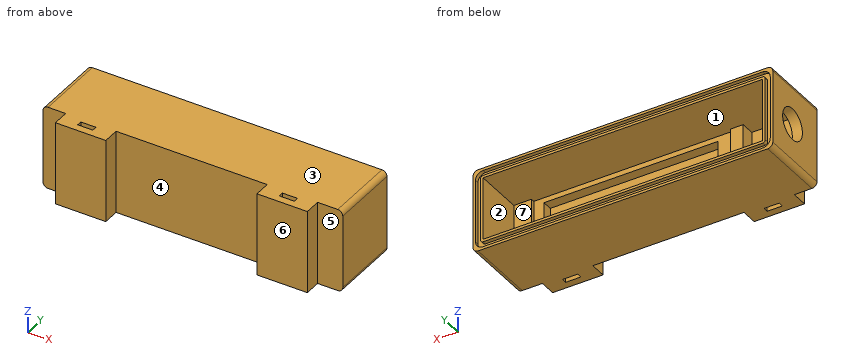
from build123d import *

# Parameters (mm, degrees)
SZKIC5_W                    = 119
SZKIC5_H                    = 33
DODANIE_WYCI_GNI_CIE3_DEPTH = 3
SZKIC6_W                    = 119
SZKIC6_H                    = 33
SZKIC6_W_2                  = 111
SZKIC6_H_2                  = 25
DODANIE_WYCI_GNI_CIE4_DEPTH = 25
SZKIC7_W                    = 91
SZKIC7_H                    = 25
SZKIC7_W_2                  = 69
SZKIC7_H_2                  = 21
DODANIE_WYCI_GNI_CIE5_DEPTH = 4
SZKIC8_W                    = 5
SZKIC8_H                    = 25
SZKIC8_W_2                  = 7
DODANIE_WYCI_GNI_CIE6_DEPTH = 1.5
SZKIC10_R                   = 6.25
WYTNIJ_WYCI_GNI_CIE1_DEPTH  = 7.5
SZKIC22_W                   = 2
SZKIC22_H                   = 3
BOSS_EXTRUDE2_DEPTH         = 20
FILLET1_R                   = 2
SKETCH2_W                   = 6
SKETCH2_H                   = 2
CUT_EXTRUDE1_DEPTH          = 33
FILLET2_R                   = 2
FILLET3_R                   = 2
CUT_EXTRUDE2_DEPTH          = 111


with BuildPart() as part:
    # Szkic5 → Dodanie-wyciągnięcie3 (new body)
    with BuildSketch(Plane(origin=(0, 0, 0), x_dir=(1, 0, 0), z_dir=(0, 1, 0))):
        Rectangle(SZKIC5_W, SZKIC5_H)
    extrude(amount=DODANIE_WYCI_GNI_CIE3_DEPTH)

    # Szkic6 → Dodanie-wyciągnięcie4 (add)
    with BuildSketch(Plane(origin=(0, 3, 0), x_dir=(1, 0, 0), z_dir=(0, 1, 0))):
        Rectangle(SZKIC6_W, SZKIC6_H)
        Rectangle(SZKIC6_W_2, SZKIC6_H_2, mode=Mode.SUBTRACT)
    extrude(amount=DODANIE_WYCI_GNI_CIE4_DEPTH)

    # Szkic7 → Dodanie-wyciągnięcie5 (add)
    with BuildSketch(Plane(origin=(0, 3, 0), x_dir=(1, 0, 0), z_dir=(0, 1, 0))):
        with Locations((10, 0)):
            Rectangle(SZKIC7_W, SZKIC7_H)
        with Locations((10, 0)):
            Rectangle(SZKIC7_W_2, SZKIC7_H_2, mode=Mode.SUBTRACT)
    extrude(amount=DODANIE_WYCI_GNI_CIE5_DEPTH)

    # Szkic8 → Dodanie-wyciągnięcie6 (add)
    with BuildSketch(Plane(origin=(0, 7, 0), x_dir=(1, 0, 0), z_dir=(0, 1, 0))):
        with Locations((-33, 0)):
            Rectangle(SZKIC8_W, SZKIC8_H)
        with Locations((52, 0)):
            Rectangle(SZKIC8_W_2, SZKIC8_H)
    extrude(amount=DODANIE_WYCI_GNI_CIE6_DEPTH)

    # Szkic10 → Wytnij-wyciągnięcie1 (cut)
    with BuildSketch(Plane(origin=(-55.5, 0, 0), x_dir=(0, 0, -1), z_dir=(1, 0, 0))):
        with Locations((0, 15.5)):
            Circle(SZKIC10_R)
    extrude(amount=-WYTNIJ_WYCI_GNI_CIE1_DEPTH, mode=Mode.SUBTRACT)

    # Wycięcie-wyciągnięcie po ścieżce1: sweep along a path in Szkic21
    with BuildLine(Plane(origin=(0, 28, 0), x_dir=(1, 0, 0), z_dir=(0, 1, 0))) as wyci_cie_wyci_gni_cie_po_cie_ce1_path:
        Line((-55.5, 14.5), (55.5, 14.5))
        ThreePointArc((55.5, 14.5), (56.914213562, 13.914213562), (57.5, 12.5))
        Line((57.5, 12.5), (57.5, -12.5))
        ThreePointArc((57.5, -12.5), (56.914213562, -13.914213562), (55.5, -14.5))
        Line((55.5, -14.5), (-55.5, -14.5))
        ThreePointArc((-55.5, -14.5), (-56.914213562, -13.914213562), (-57.5, -12.5))
        Line((-57.5, -12.5), (-57.5, 12.5))
        ThreePointArc((-57.5, 12.5), (-56.914213562, 13.914213562), (-55.5, 14.5))
    # Szkic22 → Wycięcie-wyciągnięcie po ścieżce1 (sweep, cut)
    with BuildSketch(Plane(origin=(49.5, 0, 0), x_dir=(0, 0, -1), z_dir=(1, 0, 0))):
        with Locations((14.5, 28)):
            Rectangle(SZKIC22_W, SZKIC22_H)
    sweep(path=wyci_cie_wyci_gni_cie_po_cie_ce1_path.line, mode=Mode.SUBTRACT)

    # Sketch1 → Boss-Extrude2 (add)
    with BuildSketch(Plane(origin=(49.5, 0, 0), x_dir=(0, 0, -1), z_dir=(1, 0, 0))):
        with BuildLine():
            Line((-16.5, 0), (16.5, 0))
            Line((16.5, 0), (16.5, -9))
            Line((16.5, -9), (17.83044843, -12))
            Line((17.83044843, -12), (18, -18.997946289))
            Line((18, -18.997946289), (12.5, -18.997946289))
            ThreePointArc((12.5, -18.997946289), (0, -6.497946289), (-12.5, -18.997946289))
            Line((-12.5, -18.997946289), (-18, -18.997946289))
            Line((-18, -18.997946289), (-17.83044843, -12))
            Line((-17.83044843, -12), (-16.5, -9))
            Line((-16.5, -9), (-16.5, 0))
        make_face()
    boss_extrude2 = extrude(amount=-BOSS_EXTRUDE2_DEPTH)

    # Fillet1
    fillet1_edges = [part.edges().sort_by_distance(p)[0] for p in [
        (39.5, -12, -17.83044843),
        (39.5, -18.997946289, -18),
        (39.5, -18.997946289, 18),
        (39.5, -12, 17.83044843),
        (39.5, -9, 16.5),
        (39.5, -9, -16.5),
    ]]
    fillet(fillet1_edges, radius=FILLET1_R)

    # Sketch2 → Cut-Extrude1 (cut)
    with BuildSketch(Plane.XY.offset(16.5)):
        with Locations((39.5, -2.576410505)):
            Rectangle(SKETCH2_W, SKETCH2_H)
    cut_extrude1 = extrude(amount=-CUT_EXTRUDE1_DEPTH, mode=Mode.SUBTRACT)

    # Mirror1: Boss-Extrude2 across plane
    add(boss_extrude2.mirror(Plane(origin=(-0.5, 0, 0), x_dir=(0, 0, 1), z_dir=(1, 0, 0))))

    # Mirror4: Cut-Extrude1 across plane
    add(cut_extrude1.mirror(Plane(origin=(-0.5, 0, 0), x_dir=(0, 0, 1), z_dir=(1, 0, 0))), mode=Mode.SUBTRACT)

    # Fillet2
    fillet2_edges = [part.edges().sort_by_distance(p)[0] for p in [
        (-40.5, -18.997946289, -18),
        (-40.5, -12, -17.83044843),
        (-40.5, -9, -16.5),
        (-40.5, -9, 16.5),
        (-40.5, -12, 17.83044843),
        (-40.5, -18.997946289, 18),
    ]]
    fillet(fillet2_edges, radius=FILLET2_R)

    # Fillet3
    fillet3_edges = [part.edges().sort_by_distance(p)[0] for p in [
        (59.5, 14, 16.5),
        (-59.5, 14, 16.5),
        (-59.5, 14, -16.5),
        (59.5, 14, -16.5),
    ]]
    fillet(fillet3_edges, radius=FILLET3_R)

    # Sketch3 → Cut-Extrude2 (cut, through all)
    with BuildSketch(Plane.ZY.offset(50.5)):
        Polygon((0, -6.497946289), (29.072487689, -6.497946289), (29.072487689, -24.547767437), (-22.707347074, -24.547767437), (-22.707347074, -6.497946289), align=None)
    extrude(amount=-CUT_EXTRUDE2_DEPTH, mode=Mode.SUBTRACT)


solid = part.part
Build history of the part. All positions in model axes, mm. Face numbers are marked on the shaded views. A direction names the side the tool comes from. Round coordinates to 2 decimals unless told otherwise and drop trailing zeros. Write each loop counter-clockwise with the first axis right and the second up, starting at its lowest first coordinate (ties: lowest second). Pieces come first, ordered by that corner, then holes. Notation, with made-up numbers: (44, 48) -> (102, 48) arc R8 cw to (102, 55) -> close; hole circle Ø9 at (49, 4). An arc over 180 degrees is marked (long way). Use one line per item in the form item = value.
Q1. Band-saw the part on A-A, the plane x = 17. Write the cut outline in (y, z), then the cut area to 3 significant figures.
Conclusion:
outline = (0, -16.5) -> (28, -16.5) -> (28, -15.5) -> (26.5, -15.5) -> (26.5, -13.5) -> (28, -13.5) -> (28, -12.5) -> (7, -12.5) -> (7, -10.5) -> (3, -10.5) -> (3, 10.5) -> (7, 10.5) -> (7, 12.5) -> (28, 12.5) -> (28, 13.5) -> (26.5, 13.5) -> (26.5, 15.5) -> (28, 15.5) -> (28, 16.5) -> (0, 16.5) -> close
area = 309 mm²
Q2. Drill centre lines: L1, parallel to X at y = 6, z = 8; L2, parallel to X at y = 8, z = -4; L3, parallel to Y at x = -57, z = 0. Where is each one in solid material? Low to high.
Conclusion:
L1 = -59.5 to -55.5, -35.5 to -24.5, 44.5 to 59.5
L2 = -59.5 to -55.5, -35.5 to -30.5, 48.5 to 59.5
L3 = 0 to 9.25, 21.75 to 26.5
Q3. Band-saw the part on C-C, the plane y = 15.5. Write the cut outline in (x, z), then the cut area to 3 significant figures.
Conclusion:
outline = (-59.5, -14.5) arc R2 ccw to (-57.5, -16.5) -> (57.5, -16.5) arc R2 ccw to (59.5, -14.5) -> (59.5, 14.5) arc R2 ccw to (57.5, 16.5) -> (-57.5, 16.5) arc R2 ccw to (-59.5, 14.5) -> (-59.5, 6.25) -> (-55.5, 6.25) -> (-55.5, 12.5) -> (55.5, 12.5) -> (55.5, -12.5) -> (-55.5, -12.5) -> (-55.5, -6.25) -> (-59.5, -6.25) -> close
area = 1,100 mm²
Q4. Band-saw the part on B-B, the plane z = 0. State how many separate pieces and enclosed holes the cut face has, then the cut area to 3 significant figures.
Conclusion:
separate_pieces = 2
enclosed_holes = 2
area = 843 mm²
Q5. Drop flat-ended pins along their axis: P1, Ø5, axis at x = 17, z = 6.5, coming from the +Y side; P2, Ø1, axis at y = -2.5, z = 4.5, coming from the -X side; P3, Ø3, axis at x = -27.5, z = -5, coming from the -Y side. Give the stop position or say it passes through.
Conclusion:
P1 = 3
P2 = -50.5
P3 = 0
Q6. Tool access for the marked faces 5, 6 and 7: list every direction of +Z, -Z, +X, -X, +Y, -Y with a clear straight run to the whole face (end or side of a thin tool).
Conclusion:
face_5 = +Z, -Z, +X, -Y
face_6 = +Z, -Z, +X, -X, -Y
face_7 = +Y
Q7. Two-plate mould, pull along Z, no slides. Class the marked faces 1, 2, 3 and 4: released by +Z, released by -Z, zero draft, split by the parting line, or undercut.
Conclusion:
face_1 = undercut
face_2 = undercut
face_3 = released by +Z
face_4 = zero draft
